Source: CAD feature listing. Evaluate the final solid. Frame: model axes, mm. Face numbers are marked on the shaded views. A direction names the side the tool comes from. Round coordinates to 2 decimals unless told otherwise and drop trailing zeros. Order: outer loops, then holes, each group sorted by start corner. A loop starts at its lowest first (then second) coordinate and runs counter-clockwise, first axis right, second up. Notation, with made-up numbers: M 55,63.5 L 88,63.5 A24 ccw 88,88.5 Z; hole C -5,21.25 d6. An arc over 180 degrees is marked long. Use one line per item in the form item = value. Start each with the question number.
Q1. Reachability of the marked faces 1 and 2 from +Z, -Z, +X, -X, +Y, -Y: full face, straight path, thin tool, end or side. Return the list, or none.
Q2. Section D-D (x = 12). Return the cut outline in (y, z).
Q3. Contact query for flat-ended pins moving along their axis: pin 1 (9 mm diameter, centred on x = 0, z = 28.3, fed in from +Y); pin 2 (3 mm diameter, centred on x = -2.5, z = 137.5, fed in from +Y); pin 3 (2 mm diameter, centred on x = -7, z = 93.5, fed in from -Y); pin 4 (1.5 mm diameter, centred on x = 11, z = 147, fed in from -Y). Output: stop coordinate, or through.
Q4. Section B-B (y = 0). Return the cut outline in (x, z), plus the area to 3 significant figures.
Q5. Section A-A (x = 0). Return the cut outline in (y, z), plus the area to 3 significant figures.
Q6. Section C-C (z = 141). Return the cut outline in (x, y), plus the area to 3 significant figures.
Q7. Material intervals for probe 1 along Z at (x, y) = (-3.5, -0.5); probe 2 along Z at (x, y) = (6, 9.5); probe 3 along Z at (x, y) = (1.5, -12.5), sorted ascending.
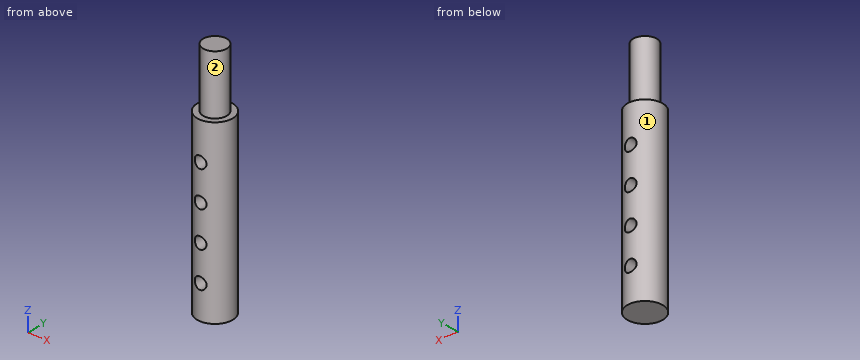
from build123d import *

# Parameters (mm, degrees)
SZKIC1_R                        = 15
DODANIE_WYCI_GNI_CIE1_DEPTH     = 150
SZKIC2_R                        = 10
DODANIE_WYCI_GNI_CIE2_DEPTH     = 50
WYTNIJ_WYCI_GNI_CIE1_DEPTH      = 70
WYTNIJ_WYCI_GNI_CIE1_DEPTH_BACK = 70
SZKIC3_R                        = 5


with BuildPart() as part:
    # Szkic1 → Dodanie-wyci_gni_cie1 (new body)
    with BuildSketch(Plane.XY):
        Circle(SZKIC1_R)
    extrude(amount=DODANIE_WYCI_GNI_CIE1_DEPTH)

    # Szkic2 → Dodanie-wyci_gni_cie2 (add)
    with BuildSketch(Plane.XY.offset(150)):
        Circle(SZKIC2_R)
    extrude(amount=DODANIE_WYCI_GNI_CIE2_DEPTH)

    # Szkic3 → Wytnij-wyci_gni_cie1 (cut, two sides: drawn at the far end of the back side and taken through both)
    with BuildSketch(Plane(origin=(0, 0, 0), x_dir=(1, 0, 0), z_dir=(0, 1, 0)).offset(-WYTNIJ_WYCI_GNI_CIE1_DEPTH_BACK)):
        with Locations(Location((0, -28.303646962, 0), (0, 0, 90))):
            Circle(SZKIC3_R)
        with Locations(Location((0, -58.303646962, 0), (0, 0, 90))):
            Circle(SZKIC3_R)
        with Locations(Location((0, -88.303646962, 0), (0, 0, 90))):
            Circle(SZKIC3_R)
        with Locations(Location((0, -118.303646962, 0), (0, 0, 90))):
            Circle(SZKIC3_R)
    extrude(amount=WYTNIJ_WYCI_GNI_CIE1_DEPTH + WYTNIJ_WYCI_GNI_CIE1_DEPTH_BACK, mode=Mode.SUBTRACT)


solid = part.part
Results list:
q1.face_1 = +Z, -Z
q1.face_2 = +Z
q2.outline = M -9,0 L 9,0 L 9,150 L -9,150 Z
q3.pin_1 = through
q3.pin_2 = 14.97
q3.pin_3 = -13.75
q3.pin_4 = -10.95
q4.outline = M -15,0 L 15,0 L 15,150 L 10,150 L 10,200 L -10,200 L -10,150 L -15,150 Z; hole C 0,28.3 d10; hole C 0,58.3 d10; hole C 0,88.3 d10; hole C 0,118.3 d10
q4.area = 5,190 mm2
q5.outline = M -15,0 L 15,0 L 15,23.3 L -15,23.3 Z; M -15,33.3 L 15,33.3 L 15,53.3 L -15,53.3 Z; M -15,63.3 L 15,63.3 L 15,83.3 L -15,83.3 Z; M -15,93.3 L 15,93.3 L 15,113.3 L -15,113.3 Z; M -15,123.3 L 15,123.3 L 15,150 L 10,150 L 10,200 L -10,200 L -10,150 L -15,150 Z
q5.area = 4,300 mm2
q6.outline = C 0,0 d30
q6.area = 707 mm2
q7.probe_1 = 0 to 24.73, 31.87 to 54.73, 61.87 to 84.73, 91.87 to 114.73, 121.87 to 200
q7.probe_2 = 0 to 150
q7.probe_3 = 0 to 23.53, 33.07 to 53.53, 63.07 to 83.53, 93.07 to 113.53, 123.07 to 150
